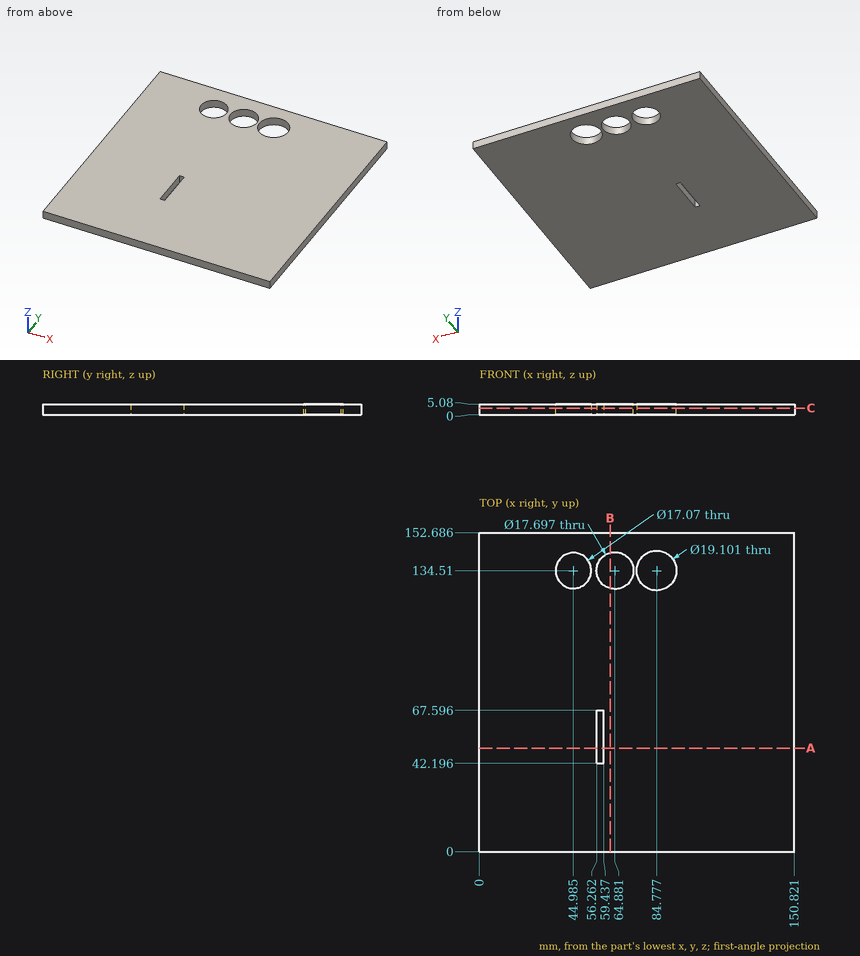
Design review of the part shown in the three views and the two pictorial views. Dimensions are in mm from the part's minimum x, y and z. Round coordinates to 2 decimals unless told otherwise and drop trailing zeros. Write each loop counter-clockwise with the first axis right and the second up, starting at its lowest first coordinate (ties: lowest second). Pieces come first, ordered by that corner, then holes.
Item 1: We need section A-A on y = 49.5. Write out the cut boundary in (x, z).
Item 2: For probe 1 along X at (y, z) = (134, 0.9) (1 decimal); probe 2 along X at (y, z) = (59, 1.7); probe 3 along Y at (x, z) = (58.5, 1.15) (1 decimal), list the stretches that pass through material, from the lowest coordinate up.
Item 3: We need section C-C on z = 3.15. State how many separate pieces and enclosed holes the cut face has, and give its area (3 significant figures).
Item 4: We need section B-B on x = 62.5. Write out the cut boundary in (y, z).
Returned:
1. outline: (0, 0) - (56.26, 0) - (56.26, 5.08) - (0, 5.08) - close; (59.44, 0) - (150.82, 0) - (150.82, 5.08) - (59.44, 5.08) - close
2. probe 1: x = 0 to 36.5, 53.5 to 56, 73.7 to 75.2, 94.3 to 150.8
2. probe 2: x = 0 to 56.26, 59.44 to 150.82
2. probe 3: y = 0 to 42.2, 67.6 to 128.4, 140.6 to 152.7
3. separate pieces: 1
3. enclosed holes: 4
3. area: 22,200 mm2
4. outline: (0, 0) - (125.99, 0) - (125.99, 5.08) - (0, 5.08) - close; (143.03, 0) - (152.69, 0) - (152.69, 5.08) - (143.03, 5.08) - close
